```python
from build123d import *

# Parameters (mm, degrees)
SKETCH1_W           = 240
SKETCH1_H           = 151
BOSS_EXTRUDE1_DEPTH = 4
SKETCH2_W           = 27
SKETCH2_H           = 45
CUT_EXTRUDE1_DEPTH  = 10
CUT_EXTRUDE10_DEPTH = 5
SKETCH15_R          = 2.5
CUT_EXTRUDE11_DEPTH = 10
SKETCH27_R          = 1.5
CUT_EXTRUDE20_DEPTH = 10
SKETCH28_R          = 2
CUT_EXTRUDE21_DEPTH = 10
SKETCH31_R          = 2
CUT_EXTRUDE24_DEPTH = 10
SKETCH32_R          = 2
CUT_EXTRUDE25_DEPTH = 10
SKETCH34_W          = 40
SKETCH34_H          = 42
CUT_EXTRUDE26_DEPTH = 10
CUT_EXTRUDE28_DEPTH = 10
SKETCH39_R          = 2
CUT_EXTRUDE31_DEPTH = 5
SKETCH40_R          = 4
SKETCH40_R_2        = 2
BOSS_EXTRUDE6_DEPTH = 5
FILLET1_R           = 3
SKETCH43_W          = 4
SKETCH43_H          = 30
BOSS_EXTRUDE8_DEPTH = 4
FILLET2_R           = 3
CUT_EXTRUDE33_DEPTH = 10
FILLET4_R           = 5
CUT_EXTRUDE34_DEPTH = 5
SKETCH46_W          = 30
SKETCH46_H          = 4
SKETCH46_W_2        = 29.8
CUT_EXTRUDE35_DEPTH = 10
SKETCH47_R          = 2
CUT_EXTRUDE36_DEPTH = 10
SKETCH48_R          = 1.995
CUT_EXTRUDE37_DEPTH = 10
SKETCH49_R          = 4
SKETCH49_R_2        = 1.868109978
SKETCH49_R_3        = 1.95
BOSS_EXTRUDE9_DEPTH = 4
SKETCH50_W          = 20
SKETCH50_H          = 4
CUT_EXTRUDE38_DEPTH = 10
SKETCH51_W          = 4
SKETCH51_H          = 20
CUT_EXTRUDE39_DEPTH = 10


with BuildPart() as part:
    # Sketch1 → Boss-Extrude1 (new body)
    with BuildSketch(Plane.XY):
        Rectangle(SKETCH1_W, SKETCH1_H)
    extrude(amount=BOSS_EXTRUDE1_DEPTH)

    # Sketch2 → Cut-Extrude1 (cut)
    with BuildSketch(Plane(origin=(0, 0, 0), x_dir=(-1, 0, 0), z_dir=(0, 0, -1))):
        with Locations((23.5, -1.5)):
            Rectangle(SKETCH2_W, SKETCH2_H)
        with Locations((-23.5, -1.5)):
            Rectangle(SKETCH2_W, SKETCH2_H)
    extrude(amount=-CUT_EXTRUDE1_DEPTH, mode=Mode.SUBTRACT)

    # Sketch14 → Cut-Extrude10 (cut)
    with BuildSketch(Plane(origin=(0, 0, 0), x_dir=(-1, 0, 0), z_dir=(0, 0, -1))):
        with BuildLine():
            Line((-56.3, 15.46), (-52.3, 15.46))
            ThreePointArc((-52.3, 15.46), (-50.3, 13.46), (-52.3, 11.46))
            Line((-52.3, 11.46), (-56.3, 11.46))
            ThreePointArc((-56.3, 11.46), (-58.3, 13.46), (-56.3, 15.46))
        make_face()
        with BuildLine():
            Line((-80.3, 15.46), (-76.3, 15.46))
            ThreePointArc((-76.3, 15.46), (-74.3, 13.46), (-76.3, 11.46))
            Line((-76.3, 11.46), (-80.3, 11.46))
            ThreePointArc((-80.3, 11.46), (-82.3, 13.46), (-80.3, 15.46))
        make_face()
        with BuildLine():
            Line((-80.3, -14.54), (-76.3, -14.54))
            ThreePointArc((-76.3, -14.54), (-74.3, -16.54), (-76.3, -18.54))
            Line((-76.3, -18.54), (-80.3, -18.54))
            ThreePointArc((-80.3, -18.54), (-82.3, -16.54), (-80.3, -14.54))
        make_face()
        with BuildLine():
            Line((-56.3, -14.54), (-52.3, -14.54))
            ThreePointArc((-52.3, -14.54), (-50.3, -16.54), (-52.3, -18.54))
            Line((-52.3, -18.54), (-56.3, -18.54))
            ThreePointArc((-56.3, -18.54), (-58.3, -16.54), (-56.3, -14.54))
        make_face()
        with BuildLine():
            Line((56.3, -14.54), (52.3, -14.54))
            ThreePointArc((52.3, -14.54), (50.3, -16.54), (52.3, -18.54))
            Line((52.3, -18.54), (56.3, -18.54))
            ThreePointArc((56.3, -18.54), (58.3, -16.54), (56.3, -14.54))
        make_face()
        with BuildLine():
            Line((80.3, -14.54), (76.3, -14.54))
            ThreePointArc((76.3, -14.54), (74.3, -16.54), (76.3, -18.54))
            Line((76.3, -18.54), (80.3, -18.54))
            ThreePointArc((80.3, -18.54), (82.3, -16.54), (80.3, -14.54))
        make_face()
        with BuildLine():
            Line((80.3, 15.46), (76.3, 15.46))
            ThreePointArc((76.3, 15.46), (74.3, 13.46), (76.3, 11.46))
            Line((76.3, 11.46), (80.3, 11.46))
            ThreePointArc((80.3, 11.46), (82.3, 13.46), (80.3, 15.46))
        make_face()
        with BuildLine():
            Line((56.3, 15.46), (52.3, 15.46))
            ThreePointArc((52.3, 15.46), (50.3, 13.46), (52.3, 11.46))
            Line((52.3, 11.46), (56.3, 11.46))
            ThreePointArc((56.3, 11.46), (58.3, 13.46), (56.3, 15.46))
        make_face()
    extrude(amount=-CUT_EXTRUDE10_DEPTH, mode=Mode.SUBTRACT)

    # Sketch15 → Cut-Extrude11 (cut)
    with BuildSketch(Plane(origin=(0, 0, 0), x_dir=(-1, 0, 0), z_dir=(0, 0, -1))):
        with Locations((-104, -27)):
            Circle(SKETCH15_R)
        with Locations((-104, 24)):
            Circle(SKETCH15_R)
        with Locations(Location((104, 24, 0), (0, 0, 180))):
            Circle(SKETCH15_R)
        with Locations(Location((104, -27, 0), (0, 0, 180))):
            Circle(SKETCH15_R)
    extrude(amount=-CUT_EXTRUDE11_DEPTH, mode=Mode.SUBTRACT)

    # Sketch27 → Cut-Extrude20 (cut)
    with BuildSketch(Plane(origin=(0, 0, 0), x_dir=(-1, 0, 0), z_dir=(0, 0, -1))):
        with Locations((-25, 25)):
            Circle(SKETCH27_R)
        with Locations((0, 25)):
            Circle(SKETCH27_R)
        with Locations((25, 25)):
            Circle(SKETCH27_R)
    extrude(amount=-CUT_EXTRUDE20_DEPTH, mode=Mode.SUBTRACT)

    # Sketch28 → Cut-Extrude21 (cut)
    with BuildSketch(Plane.XY.offset(4)):
        with Locations((112, -52.5)):
            Circle(SKETCH28_R)
        with Locations((65, -52.5)):
            Circle(SKETCH28_R)
        with Locations((-65, -52.5)):
            Circle(SKETCH28_R)
        with Locations((-112, -52.5)):
            Circle(SKETCH28_R)
    extrude(amount=-CUT_EXTRUDE21_DEPTH, mode=Mode.SUBTRACT)

    # Sketch31 → Cut-Extrude24 (cut)
    with BuildSketch(Plane(origin=(0, 0, 0), x_dir=(-1, 0, 0), z_dir=(0, 0, -1))):
        with Locations((72.345744872, -69.339745962)):
            Circle(SKETCH31_R)
        with Locations(Location((-72.345744872, -69.339745962, 0), (0, 0, 180))):
            Circle(SKETCH31_R)
    extrude(amount=-CUT_EXTRUDE24_DEPTH, mode=Mode.SUBTRACT)

    # Sketch32 → Cut-Extrude25 (cut)
    with BuildSketch(Plane(origin=(0, 0, 0), x_dir=(-1, 0, 0), z_dir=(0, 0, -1))):
        with Locations((52.005844325, -34.1100048)):
            Circle(SKETCH32_R)
        with Locations(Location((-52.005844325, -34.1100048, 0), (0, 0, 180))):
            Circle(SKETCH32_R)
    extrude(amount=-CUT_EXTRUDE25_DEPTH, mode=Mode.SUBTRACT)

    # Sketch34 → Cut-Extrude26 (cut)
    with BuildSketch(Plane(origin=(0, 0, 0), x_dir=(-1, 0, 0), z_dir=(0, 0, -1))):
        with Locations((-100, 54.5)):
            Rectangle(SKETCH34_W, SKETCH34_H)
    extrude(amount=-CUT_EXTRUDE26_DEPTH, mode=Mode.SUBTRACT)

    # Sketch36 → Cut-Extrude28 (cut)
    with BuildSketch(Plane(origin=(0, 0, 0), x_dir=(-1, 0, 0), z_dir=(0, 0, -1))):
        with BuildLine():
            Line((102, 40.5), (102, 55.5))
            ThreePointArc((102, 55.5), (107, 60.5), (112, 55.5))
            Line((112, 55.5), (112, 40.5))
            ThreePointArc((112, 40.5), (107, 35.5), (102, 40.5))
        make_face()
    extrude(amount=-CUT_EXTRUDE28_DEPTH, mode=Mode.SUBTRACT)

    # Sketch39 → Cut-Extrude31 (cut)
    with BuildSketch(Plane(origin=(0, 0, 0), x_dir=(-1, 0, 0), z_dir=(0, 0, -1))):
        with Locations((107.8, 73)):
            Circle(SKETCH39_R)
    extrude(amount=-CUT_EXTRUDE31_DEPTH, mode=Mode.SUBTRACT)

    # Sketch40 → Boss-Extrude6 (add)
    with BuildSketch(Plane(origin=(0, 0, 0), x_dir=(-1, 0, 0), z_dir=(0, 0, -1))):
        with Locations((107.8, 73)):
            Circle(SKETCH40_R)
        with Locations((107.8, 73)):
            Circle(SKETCH40_R_2, mode=Mode.SUBTRACT)
    extrude(amount=-BOSS_EXTRUDE6_DEPTH)

    # Fillet1
    fillet1_edges = [part.edges().sort_by_distance(p)[0] for p in [
        (80, 33.5, 2),
    ]]
    fillet(fillet1_edges, radius=FILLET1_R)

    # Sketch43 → Boss-Extrude8 (add)
    with BuildSketch(Plane(origin=(0, 0, 0), x_dir=(-1, 0, 0), z_dir=(0, 0, -1))):
        with Locations((-122, 3.5)):
            Rectangle(SKETCH43_W, SKETCH43_H)
        with Locations((122, 24.5)):
            Rectangle(SKETCH43_W, SKETCH43_H)
    extrude(amount=-BOSS_EXTRUDE8_DEPTH)

    # Fillet2
    fillet2_edges = [part.edges().sort_by_distance(p)[0] for p in [
        (80, 75.5, 2),
    ]]
    fillet(fillet2_edges, radius=FILLET2_R)

    # Sketch44 → Cut-Extrude33 (cut)
    with BuildSketch(Plane(origin=(0, 0, 0), x_dir=(-1, 0, 0), z_dir=(0, 0, -1))):
        Polygon((-98.317208235, -75.501625548), (-120, -62.983059886), (-120, -75.5), align=None)
        Polygon((98.317208235, -75.501625548), (120, -62.983059886), (120, -75.5), align=None)
    extrude(amount=-CUT_EXTRUDE33_DEPTH, mode=Mode.SUBTRACT)

    # Fillet4
    fillet4_edges = [part.edges().sort_by_distance(p)[0] for p in [
        (98.320023767, -75.5, 2),
        (120, -62.983059886, 2),
        (-98.320023767, -75.5, 2),
        (-120, -62.983059886, 2),
    ]]
    fillet(fillet4_edges, radius=FILLET4_R)

    # Sketch45 → Cut-Extrude34 (cut)
    with BuildSketch(Plane(origin=(0, 0, 0), x_dir=(-1, 0, 0), z_dir=(0, 0, -1))):
        with BuildLine():
            Line((-62, 65.5), (-62, 50.5))
            ThreePointArc((-62, 50.5), (-67, 45.5), (-72, 50.5))
            Line((-72, 50.5), (-72, 65.5))
            ThreePointArc((-72, 65.5), (-67, 70.5), (-62, 65.5))
        make_face()
    extrude(amount=-CUT_EXTRUDE34_DEPTH, mode=Mode.SUBTRACT)

    # Sketch46 → Cut-Extrude35 (cut)
    with BuildSketch(Plane(origin=(0, 0, 0), x_dir=(-1, 0, 0), z_dir=(0, 0, -1))):
        with Locations((0, -53.5)):
            Rectangle(SKETCH46_W, SKETCH46_H)
        with Locations((-0.1, -38.5)):
            Rectangle(SKETCH46_W_2, SKETCH46_H)
        with Locations((-0.1, 35.5)):
            Rectangle(SKETCH46_W_2, SKETCH46_H)
        with Locations((0, 67.5)):
            Rectangle(SKETCH46_W_2, SKETCH46_H)
    extrude(amount=-CUT_EXTRUDE35_DEPTH, mode=Mode.SUBTRACT)

    # Sketch47 → Cut-Extrude36 (cut)
    with BuildSketch(Plane(origin=(0, 0, 0), x_dir=(-1, 0, 0), z_dir=(0, 0, -1))):
        with Locations((29.39999999, 35.5)):
            Circle(SKETCH47_R)
        with Locations((-29.39999999, 35.5)):
            Circle(SKETCH47_R)
        with Locations((-43.4, 67.5)):
            Circle(SKETCH47_R)
        with Locations((43.4, 67.5)):
            Circle(SKETCH47_R)
        with Locations((29.39999999, -38.5)):
            Circle(SKETCH47_R)
        with Locations((-29.39999999, -38.5)):
            Circle(SKETCH47_R)
        with Locations((43, -53.5)):
            Circle(SKETCH47_R)
        with Locations((-43, -53.5)):
            Circle(SKETCH47_R)
    extrude(amount=-CUT_EXTRUDE36_DEPTH, mode=Mode.SUBTRACT)

    # Sketch48 → Cut-Extrude37 (cut)
    with BuildSketch(Plane(origin=(0, 0, 0), x_dir=(-1, 0, 0), z_dir=(0, 0, -1))):
        with Locations((-39.8, -73.5)):
            Circle(SKETCH48_R)
        with Locations((39.8, -73.5)):
            Circle(SKETCH48_R)
    extrude(amount=-CUT_EXTRUDE37_DEPTH, mode=Mode.SUBTRACT)

    # Sketch49 → Boss-Extrude9 (add)
    # profile 1 of 2: a face of its own
    with BuildSketch(Plane(origin=(0, 0, 0), x_dir=(-1, 0, 0), z_dir=(0, 0, -1))):
        with Locations((-39.8, -73.5)):
            Circle(SKETCH49_R)
        with Locations((-39.8, -73.5)):
            Circle(SKETCH49_R_2, mode=Mode.SUBTRACT)
    # profile 2 of 2: a face of its own
    with BuildSketch(Plane(origin=(0, 0, 0), x_dir=(-1, 0, 0), z_dir=(0, 0, -1))):
        with Locations((39.8, -73.5)):
            Circle(SKETCH49_R)
        with Locations((39.8, -73.5)):
            Circle(SKETCH49_R_3, mode=Mode.SUBTRACT)
    extrude(amount=-BOSS_EXTRUDE9_DEPTH)

    # Sketch50 → Cut-Extrude38 (cut)
    with BuildSketch(Plane.XY.offset(4)):
        with Locations((-61, 23)):
            Rectangle(SKETCH50_W, SKETCH50_H)
    extrude(amount=-CUT_EXTRUDE38_DEPTH, mode=Mode.SUBTRACT)

    # Sketch51 → Cut-Extrude39 (cut)
    with BuildSketch(Plane(origin=(0, 0, 0), x_dir=(-1, 0, 0), z_dir=(0, 0, -1))):
        with Locations((-34, 53.25)):
            Rectangle(SKETCH51_W, SKETCH51_H)
        with Locations((34, 53.25)):
            Rectangle(SKETCH51_W, SKETCH51_H)
    extrude(amount=-CUT_EXTRUDE39_DEPTH, mode=Mode.SUBTRACT)


solid = part.part
```
The listing builds one solid part. Answer for the finished solid, in the listing's coordinates (mm). A direction names the side the tool comes from. Round coordinates to 2 decimals unless told otherwise and drop trailing zeros. Order: outer loops, then holes, each group sorted by start corner. A loop starts at its lowest first (then second) coordinate and runs counter-clockwise, first axis right, second up. Notation, with made-up numbers: (0, -33.75) -> (31, -33.75) arc R11 ccw to (31, -14.75) -> close; hole circle Ø2 at (16.25, -17.75). An arc over 180 degrees is marked (long way). Answer as CSV lines item,"result". Start each with the question number.
(1) Find the intervals of material crossed by probe 1 along Y at (x, z) = (-29, 3.5); probe 2 along Y at (x, z) = (13, 1.45); probe 3 along Y at (x, z) = (8.5, 0.65), in increasing order. Write a range as from..to.
(2) A tool of negligible diameter and unlimited length cuts with its end or side. For faces 1 (the face through (-107.279, 76.966, 3.021)), 2 (the face through (-109, 75, 5)), 3 (the face through (-107.1, 35.5, 2)), from which of +Z, -Z, +X, -X, +Y, -Y can it reach the whole face along a straight path? Write none if from no direction.
(3) The part is cut by section A-A (y = -8). Determine the outline of the cut face in (x, z), then the cut area to 3 significant figures.
(4) The part is cut by section B-B (y = 58). Determine the outline of the cut face in (x, z), then the cut area to 3 significant figures.
(5) Flat-ended cylindrical pins translate along their axes: pin 1 Ø1.5 at (x, y) = (42.5, -25) entering from -Z; pin 2 Ø1.2 at (y, z) = (67, 2.5) entering from +X; pin 3 Ø3 at (y, z) = (-54, 3) entering from -X; pin 4 Ø3 at (x, z) = (2.5, 2) entering from -Y. Find the tip coordinate at first contact, or state that the pin passes through.
(6) The part is cut by section C-C (z = 3.15). Count the separate pieces of the cut face and the enclosed holes in it, then the cut area to 3 significant figures.
Evaluation:
1,probe 1,"-75.5..-40.46, -36.54..-24, 21..33.54, 37.46..75.5"
1,probe 2,"-75.5..-55.5, -51.5..-40.5, -36.5..-24, 21..33.5, 37.5..65.5, 69.5..75.5"
1,probe 3,"-75.5..-55.5, -51.5..-40.5, -36.5..33.5, 37.5..65.5, 69.5..75.5"
2,face 1,"+Z"
2,face 2,"+Z, +X, -X, +Y, -Y"
2,face 3,"+Z, -Z"
3,outline,"(-120, 0) -> (-37, 0) -> (-37, 4) -> (-120, 4) -> close; (-10, 0) -> (10, 0) -> (10, 4) -> (-10, 4) -> close; (37, 0) -> (124, 0) -> (124, 4) -> (37, 4) -> close"
3,area,"760 mm²"
4,outline,"(-120, 0) -> (-111.33, 0) -> (-111.33, 4) -> (-120, 4) -> close; (-102.67, 0) -> (-36, 0) -> (-36, 4) -> (-102.67, 4) -> close; (-32, 0) -> (32, 0) -> (32, 4) -> (-32, 4) -> close; (36, 0) -> (62, 0) -> (62, 4) -> (36, 4) -> close; (72, 0) -> (80, 0) -> (80, 4) -> (72, 4) -> close"
4,area,"693 mm²"
5,pin 1,"z = 0"
5,pin 2,"x = 80"
5,pin 3,"x = -120"
5,pin 4,"y = -75.5"
6,separate pieces,"1"
6,enclosed holes,"45"
6,area,"30,400 mm²"
